from build123d import *

# Parameters (mm, degrees)
EXTRUDE_1_DEPTH        = 20
FILLET_1_R             = 10
HOLE_WIZARD_M3_1_D     = 3.4
HOLE_WIZARD_M3_1_DEPTH = 20
HOLE_WIZARD_M3_1_TIP   = 1.021463052
HOLE_WIZARD_M4_1_D     = 4.5
HOLE_WIZARD_M4_1_DEPTH = 20
HOLE_WIZARD_M4_1_TIP   = 1.351936393
HOLE_WIZARD_M3_2_D     = 3.4
FILLET_2_R             = 1
SKETCH_8_R             = 3.5
CUT_EXTRUDE_1_DEPTH    = 10


with BuildPart() as part:
    # 草图1 → 凸台-拉伸1 (new body)
    with BuildSketch(Plane(origin=(0, 0, 0), x_dir=(0, 0, -1), z_dir=(1, 0, 0))):
        Polygon((0, 0), (0, 40), (55, 40), (55, 0), (60, 0), (60, 45), (-5, 45), (-5, 0), align=None)
    extrude(amount=EXTRUDE_1_DEPTH)

    # 圆角1
    fillet_1_edges = [part.edges().sort_by_distance(p)[0] for p in [
        (0, 0, -57.5),
        (20, 0, -57.5),
        (0, 0, 2.5),
        (20, 0, 2.5),
    ]]
    fillet(fillet_1_edges, radius=FILLET_1_R - 0.0001)  # a hair under: the kernel refuses the full size

    # M3 间隙孔1
    with Locations(Plane.XY.offset(-55)):
        with Locations((10, 3), (10, 17), (3, 10), (17, 10)):
            Hole(HOLE_WIZARD_M3_1_D / 2, depth=HOLE_WIZARD_M3_1_DEPTH)
            with Locations((0, 0, -(HOLE_WIZARD_M3_1_DEPTH + HOLE_WIZARD_M3_1_TIP / 2))):  # 118° drill point
                Cone(0, HOLE_WIZARD_M3_1_D / 2, HOLE_WIZARD_M3_1_TIP, mode=Mode.SUBTRACT)

    # M4 间隙孔1
    with Locations(Plane(origin=(0, 0, 0), x_dir=(-1, 0, 0), z_dir=(0, 0, -1))):
        with Locations((-10, 10)):
            Hole(HOLE_WIZARD_M4_1_D / 2, depth=HOLE_WIZARD_M4_1_DEPTH)
            with Locations((0, 0, -(HOLE_WIZARD_M4_1_DEPTH + HOLE_WIZARD_M4_1_TIP / 2))):  # 118° drill point
                Cone(0, HOLE_WIZARD_M4_1_D / 2, HOLE_WIZARD_M4_1_TIP, mode=Mode.SUBTRACT)

    # M3 间隙孔2 (through all)
    with Locations(Plane(origin=(0, 45, 0), x_dir=(1, 0, 0), z_dir=(0, 1, 0))):
        with Locations((15, 17), (10, 22), (5, 17), (10, 12)):
            Hole(HOLE_WIZARD_M3_2_D / 2)

    # 圆角2
    fillet_2_edges = [part.edges().sort_by_distance(p)[0] for p in [
        (0, 24.99995, -55),
        (0, 40, -27.5),
        (20, 40, -27.5),
        (10, 45, 5),
        (10, 45, -60),
        (10, 40, -55),
        (20, 24.99995, -55),
        (0, 27.49995, -60),
        (20, 27.49995, -60),
        (17.071097101, 2.928902899, -60),
        (2.928902899, 2.928902899, -60),
        (0, 24.99995, 0),
        (20, 45, -27.5),
        (17.071097101, 2.928902899, -55),
        (2.928902899, 2.928902899, -55),
        (20, 24.99995, 0),
        (20, 27.49995, 5),
        (17.071097101, 2.928902899, 0),
        (2.928902899, 2.928902899, 0),
        (17.071097101, 2.928902899, 5),
        (2.928902899, 2.928902899, 5),
        (0, 27.49995, 5),
        (0, 45, -27.5),
    ]]
    fillet(fillet_2_edges, radius=FILLET_2_R)

    # 草图8 → 切除-拉伸1 (cut)
    with BuildSketch(Plane(origin=(0, 0, -60), x_dir=(-1, 0, 0), z_dir=(0, 0, -1))):
        with Locations((-10, 10)):
            Circle(SKETCH_8_R)
    extrude(amount=-CUT_EXTRUDE_1_DEPTH, mode=Mode.SUBTRACT)


solid = part.part
The listing builds one solid part. Answer for the finished solid, in the listing's coordinates (mm). A direction names the side the tool comes from. Give positions to 0.01 mm unless a question says otherwise; leave off trailing zeros. Write each loop counter-clockwise with the first axis right and the second up, starting at its lowest first coordinate (ties: lowest second). Pieces come first, ordered by that corner, then holes.
1) Section B-B (z = -12) is taken. Write down the section's boundary in (x, y).
2) Given P1, Ø5, axis at x = 9.5, z = -45.5, coming from the -Y side; P2, Ø3, axis at x = 10, y = 17, coming from the -Z side, each flat-ended and moving along its own axis, determine where each tip first touches the part or whether it passes through.
3) Section A-A (y = 17) is taken. Write down the section's boundary in (x, z).
4) For a pull along Z with two mould halves and no side action, classify faces 4 (the face through (10, 27, -60)), 5 (the face through (8.38, 3.51, -57.54)), 6 (the face through (9.086, 42.465, -13.433)) as pulls with the +Z half, pulls with the -Z half, needs draft (parallel to the pull), parting line crosses it, or undercut.
5) Section D-D (z = -23) is taken. Write down the section's boundary in (x, y).
6) Find the intervals of material crossed by L1, parallel to Z at x = 10, y = 41.85; L2, parallel to Y at x = 10, z = -58.75; L3, parallel to X at y = 42.55, z = -17, in increasing order.
7) A tool of negligible diameter and unlimited length cuts with its end or side. For faces 1 (the face through (1.43, 9.35, -57.54)), 2 (the face through (10, 45, -28)), 3 (the face through (10, 20, -55)), from which of +Z, -Z, +X, -X, +Y, -Y can it reach the whole face along a straight path? Write none if from no direction.
8) Section C-C (y = 22.5) is taken. Write down the section's boundary in (x, z), and give its area (3 significant figures).
Response:
1. outline: (0, 41) arc R1 ccw to (1, 40) - (8.3, 40) - (8.3, 45) - (1, 45) arc R1 ccw to (0, 44) - close; (11.7, 40) - (19, 40) arc R1 ccw to (20, 41) - (20, 44) arc R1 ccw to (19, 45) - (11.7, 45) - close
2. P1: stops at y = 40
2. P2: stops at z = 0
3. outline: (0, -59) arc R1 ccw to (1, -60) - (8.3, -60) - (8.3, -55) - (1, -55) arc R1 ccw to (0, -56) - close; (0, 1) arc R1 ccw to (1, 0) - (19, 0) arc R1 ccw to (20, 1) - (20, 4) arc R1 ccw to (19, 5) - (1, 5) arc R1 ccw to (0, 4) - close; (11.7, -60) - (19, -60) arc R1 ccw to (20, -59) - (20, -56) arc R1 ccw to (19, -55) - (11.7, -55) - close
4. face 4: pulls with the -Z half
4. face 5: needs draft
4. face 6: undercut
5. outline: (0, 41) arc R1 ccw to (1, 40) - (8.63, 40) - (8.63, 45) - (1, 45) arc R1 ccw to (0, 44) - close; (11.37, 40) - (19, 40) arc R1 ccw to (20, 41) - (20, 44) arc R1 ccw to (19, 45) - (11.37, 45) - close
6. L1: z = -60 to -23.7, -20.3 to -13.7, -10.3 to 5
6. L2: y = 0 to 1.3, 4.7 to 6.5, 13.5 to 15.3, 18.7 to 45
6. L3: x = 0 to 3.3, 6.7 to 13.3, 16.7 to 20
7. face 1: -Z
7. face 2: +Z, -Z, +X, -X, +Y
7. face 3: +X, -X, -Y
8. outline: (0, -59) arc R1 ccw to (1, -60) - (19, -60) arc R1 ccw to (20, -59) - (20, -56) arc R1 ccw to (19, -55) - (1, -55) arc R1 ccw to (0, -56) - close; (0, 1) arc R1 ccw to (1, 0) - (19, 0) arc R1 ccw to (20, 1) - (20, 4) arc R1 ccw to (19, 5) - (1, 5) arc R1 ccw to (0, 4) - close
8. area: 198 mm2
